Design review of the part built by this model. Coordinates are the model's own, in mm. A direction names the side the tool comes from. Coordinates: 2 decimals unless noted, no trailing zeros. Write each loop counter-clockwise with the first axis right and the second up, starting at its lowest first coordinate (ties: lowest second). Pieces come first, ordered by that corner, then holes.
Q1. Take a section at A-A, the plane z = 0. Write out the cut boundary in (x, y).
Q2. Take a section at B-B, the plane y = 0. Write out the cut boundary in (x, z), plus the area to 3 significant figures.
Q3. For L1, parallel to Z at x = 3, y = 0; L2, parallel to X at y = -7, z = 5.5; L3, parallel to X at y = 10.5, z = 8.5, list the stretches that pass through material, from the lowest coordinate up.
Q4. Take a section at C-C, the plane y = -16. Write out the cut boundary in (x, z).
Q5. Take a section at D-D, the plane z = -10.5. Write out the cut boundary in (x, y).
Q6. For faces 1 (the cylindrical face through (2.96, -12.23, 6.84)), 2 (the flat face through (23, 14, -11)), 3 (the flat face through (-22, -7, 0)), list the 3-axis set-ups (+Z, -Z, +X, -X, +Y, -Y) from which the entire face can be reached by the end or side of a thin tool; tool diameter is ignored.
Q7. The part is to be moulded in two halves that separate along Y. For faces 4 (the flat face through (-6, -4, -1)), 5 (the cylindrical face through (-13.89, -9.77, -1.15)), 6 (the cylindrical face through (2.958, -0.806, 16.765)), say which applies: released by +Y, released by -Y, zero draft, split by the parting line, or undercut.
Q8. For pin 1 Ø2.5 at (y, z) = (-0.5, -16) entering from -X; pin 2 Ø1.8 at (y, z) = (-13.42, 7.75) entering from -X; pin 3 Ø1.5 at (x, z) = (-14, -5) entering from +Y; pin 4 Ø5 at (x, y) = (9, 9.5) entering from +Z, all flat-tipped, find the tip position at first contact; note any pin that passes through.
from build123d import *

# Parameters (mm, degrees)
SKETCH3_R           = 3
BOSS_EXTRUDE1_DEPTH = 22
SKETCH3_3_R         = 6
BOSS_EXTRUDE2_DEPTH = 6
SKETCH4_R           = 1.5
CUT_EXTRUDE1_DEPTH  = 6


with BuildPart() as part:
    # Sketch2 → Revolve1 (revolve)
    with BuildSketch(Plane.XY):
        Polygon((0, 0), (0, 18.4), (23, 18.4), (23, 17.4), (53.7, 17.4), (53.7, 0), align=None)
    revolve(axis=Axis((53.7, 0, 0), (-1, 0, 0)))

    # Sketch3 → Boss-Extrude1 (add)
    with BuildSketch(Plane.ZY):
        with Locations(Location((0, -7, 0), (0, 0, 270))):
            Circle(SKETCH3_R)
    extrude(amount=BOSS_EXTRUDE1_DEPTH)

    # Sketch3_3 → Boss-Extrude2 (add)
    with BuildSketch(Plane.ZY):
        with Locations(Location((0, -7, 0), (0, 0, 270))):
            Circle(SKETCH3_3_R)
    extrude(amount=BOSS_EXTRUDE2_DEPTH)

    # Sketch4 → Cut-Extrude1 (cut)
    with BuildSketch(Plane.ZY):
        with Locations(Location((15.5, 0, 0), (0, 0, 270))):
            Circle(SKETCH4_R)
        with Locations(Location((7.75, -13.423393759, 0), (0, 0, 270))):
            Circle(SKETCH4_R)
        with Locations(Location((-7.75, -13.423393759, 0), (0, 0, 270))):
            Circle(SKETCH4_R)
        with Locations(Location((-15.5, 0, 0), (0, 0, 270))):
            Circle(SKETCH4_R)
        with Locations(Location((-7.75, 13.423393759, 0), (0, 0, 270))):
            Circle(SKETCH4_R)
        with Locations(Location((7.75, 13.423393759, 0), (0, 0, 270))):
            Circle(SKETCH4_R)
    extrude(amount=-CUT_EXTRUDE1_DEPTH, mode=Mode.SUBTRACT)


solid = part.part
Responses:
1. outline: (-22, -10) - (-6, -10) - (-6, -13) - (0, -13) - (0, -18.4) - (23, -18.4) - (23, -17.4) - (53.7, -17.4) - (53.7, 17.4) - (23, 17.4) - (23, 18.4) - (0, 18.4) - (0, -1) - (-6, -1) - (-6, -4) - (-22, -4) - close
2. outline: (0, -18.4) - (23, -18.4) - (23, -17.4) - (53.7, -17.4) - (53.7, 17.4) - (23, 17.4) - (23, 18.4) - (0, 18.4) - (0, 17) - (6, 17) - (6, 14) - (0, 14) - (0, -14) - (6, -14) - (6, -17) - (0, -17) - close
2. area: 1,880 mm2
3. L1: z = -18.4 to -17, -14 to 14, 17 to 18.4
3. L2: x = -6 to 53.7
3. L3: x = 0 to 53.7
4. outline: (0, -9.09) - (23, -9.09) - (23, -6.84) - (53.7, -6.84) - (53.7, 6.84) - (23, 6.84) - (23, 9.09) - (0, 9.09) - close
5. outline: (0, -15.11) - (23, -15.11) - (23, -13.87) - (53.7, -13.87) - (53.7, 13.87) - (23, 13.87) - (23, 15.11) - (0, 15.11) - close
6. face 1: -X
6. face 2: +X
6. face 3: +Z, -Z, -X, +Y, -Y
7. face 4: zero draft
7. face 5: split by the parting line
7. face 6: undercut
8. pin 1: stops at x = 0
8. pin 2: stops at x = 6
8. pin 3: passes through
8. pin 4: stops at z = 17.02
